Read the model definition and answer for the solid it produces. Units are mm, in the model's axes. Face numbers are marked on the shaded views. A direction names the side the tool comes from. Give positions to 0.01 mm unless a question says otherwise; leave off trailing zeros. Order: outer loops, then holes, each group sorted by start corner. A loop starts at its lowest first (then second) coordinate and runs counter-clockwise, first axis right, second up. Notation, with made-up numbers: (-15, 56) - (-4, 56) arc R35 ccw to (-4, 89) - close; hole circle Ø5 at (14.25, 83.5). An arc over 180 degrees is marked (long way). Write each question's results on one line, items separated by ' | '. Start each with the question number.
Q1. Find the intervals of material crossed by line 1 along Y through (x, z) = (5, 11); line 2 along X through (y, z) = (-0.3, 0); line 3 along X through (y, z) = (-0.15, -13.25), in increasing order. Write a range as from..to.
Q2. Find section B-B on x = 11.25. Give the vertices of the cut face in (y, z), and give its area (3 significant figures).
Q3. Flat-ended cylindrical pins translate along their axes: P1, Ø13, axis at y = 20.5, z = -6.5, coming from the +X side; P2, Ø10, axis at x = 10.5, z = 4, coming from the +Y side. Find the tip coordinate at first contact, or state that the pin passes through.
Q4. Find section A-A on z = 0. Give the vertices of the cut face in (x, y), and give its area (3 significant figures).
Q5. A tool of negligible diameter and unlimited length cuts with its end or side. For the marked faces 1 and 2, from which of +Z, -Z, +X, -X, +Y, -Y can it reach the whole face along a straight path? Write none if from no direction.
Q6. Find section C-C on z = -13.25. Give the vertices of the cut face in (x, y).
Q7. Find section D-D on y = 19. Give the vertices of the cut face in (x, z).
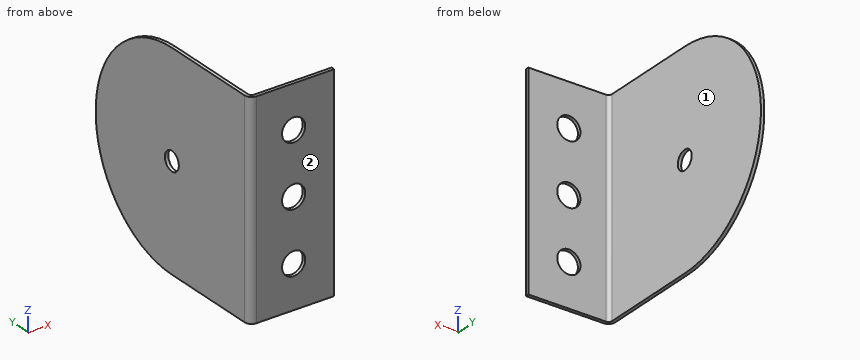
from build123d import *

# Parameters (mm, degrees)
SKETCH1_R                  = 2.5
SKETCH1_R_2                = 2.06
BASE_FLANGE3_DEPTH         = 0.7366
SKETCHED_START             = -43
SKETCHED_BEND1_OUTLINE_W   = 0.7366
SKETCHED_BEND1_OUTLINE_H   = 45
SKETCHED_BEND1_DEPTH       = 44.914756568
SKETCHED_START_2           = 2.495963432
SKETCHED_BEND1_2_OUTLINE_R = 2.06
SKETCHED_BEND1_2_DEPTH     = 0.004036568
SKETCHED_START_3           = 1.7634
SKETCHED_BEND1_3_OUTLINE_R = 2.06
SKETCHED_BEND1_3_DEPTH     = 1.4732
SKETCHED_START_4           = -23
SKETCHED_BEND1_4_DEPTH     = 46


with BuildPart() as part:
    # Base-Flange3: sheet metal written as solids
    # Sketch1 → Base-Flange3 (new body)
    with BuildSketch(Plane(origin=(0, 0, 0), x_dir=(1, 0, 0), z_dir=(0, 1, 0))):
        with BuildLine():
            Line((-20, 22.5), (20, 22.5))
            Line((20, 22.5), (20, -22.5))
            Line((20, -22.5), (-20, -22.5))
            ThreePointArc((-20, -22.5), (-42.5, 0), (-20, 22.5))
        make_face()
        with Locations(Location((11.25, -13.25, 0), (0, 0, 270))):
            Circle(SKETCH1_R, mode=Mode.SUBTRACT)
        with Locations(Location((11.25, 13.25, 0), (0, 0, 270))):
            Circle(SKETCH1_R, mode=Mode.SUBTRACT)
        with Locations(Location((11.25, 0, 0), (0, 0, 270))):
            Circle(SKETCH1_R, mode=Mode.SUBTRACT)
        with Locations(Location((-20, 0, 0), (0, 0, 270))):
            Circle(SKETCH1_R_2, mode=Mode.SUBTRACT)
    extrude(amount=-BASE_FLANGE3_DEPTH)

    # Sketched Bend1: read off the stored shape, not the designer's step
    # Sketched Bend1 outline → Sketched Bend1 (cut)
    with BuildSketch(Plane.YZ.offset(SKETCHED_START)):
        with Locations((-0.3683, 0)):
            Rectangle(SKETCHED_BEND1_OUTLINE_W, SKETCHED_BEND1_OUTLINE_H)
    extrude(amount=SKETCHED_BEND1_DEPTH, mode=Mode.SUBTRACT)

    # Sketched Bend1 2 outline → Sketched Bend1 2 (add)
    with BuildSketch(Plane.YZ.offset(SKETCHED_START_2)):
        with BuildLine():
            ThreePointArc((22.237627139, -22.5), (44.737627139, 0), (22.237627139, 22.5))
            Line((22.237627139, 22.5), (0, 22.5))
            Line((0, 22.5), (0, -22.5))
            Line((0, -22.5), (22.237627139, -22.5))
        make_face()
        with Locations((22.237627139, 0)):
            Circle(SKETCHED_BEND1_2_OUTLINE_R, mode=Mode.SUBTRACT)
    extrude(amount=SKETCHED_BEND1_2_DEPTH)

    # Sketched Bend1 3 outline → Sketched Bend1 3 (add)
    with BuildSketch(Plane.YZ.offset(SKETCHED_START_3)):
        with BuildLine():
            ThreePointArc((22.237627139, -22.5), (44.737627139, 0), (22.237627139, 22.5))
            Line((22.237627139, 22.5), (0, 22.5))
            Line((0, 22.5), (0, -22.5))
            Line((0, -22.5), (22.237627139, -22.5))
        make_face()
        with Locations((22.237627139, 0)):
            Circle(SKETCHED_BEND1_3_OUTLINE_R, mode=Mode.SUBTRACT)
    extrude(amount=SKETCHED_BEND1_3_DEPTH)

    # Sketched Bend1 4 outline → Sketched Bend1 4 (cut)
    with BuildSketch(Plane.XY.offset(SKETCHED_START_4)):
        with BuildLine():
            Line((2.5, 46), (2.5, 0.7366))
            ThreePointArc((2.5, 0.7366), (2.715745145, 0.215745145), (3.2366, 0))
            Line((3.2366, 0), (3.2366, 46))
            Line((3.2366, 46), (2.5, 46))
        make_face()
        with BuildLine():
            Line((1.7634, 0.7366), (1.763399995, 46))
            Line((1.763399995, 46), (0, 46))
            Line((0, 46), (0, 0))
            Line((0, 0), (1.914756568, 0))
            Line((1.914756568, 0), (1.914756568, -2))
            Line((1.914756568, -2), (5, -2))
            Line((5, -2), (5, -0.7366))
            Line((5, -0.7366), (3.2366, -0.7366))
            ThreePointArc((3.2366, -0.7366), (2.19489029, -0.30510971), (1.7634, 0.7366))
        make_face()
    extrude(amount=SKETCHED_BEND1_4_DEPTH, mode=Mode.SUBTRACT)


solid = part.part
Working result:
1) line 1: -0.74..0 | line 2: 2.19..8.75, 13.75..20 | line 3: 2.06..8.75, 13.75..20
2) outline: (-0.74, -22.5) - (0, -22.5) - (0, -15.75) - (-0.74, -15.75) - close; (-0.74, -10.75) - (0, -10.75) - (0, -2.5) - (-0.74, -2.5) - close; (-0.74, 2.5) - (0, 2.5) - (0, 10.75) - (-0.74, 10.75) - close; (-0.74, 15.75) - (0, 15.75) - (0, 22.5) - (-0.74, 22.5) - close | area: 22.1 mm²
3) P1: x = 2.5 | P2: y = 0
4) outline: (1.76, 0.74) arc R1.47 ccw to (3.24, -0.74) - (8.75, -0.74) - (8.75, 0) - (3.24, 0) arc R0.74 cw to (2.5, 0.74) - (2.5, 20.18) - (1.76, 20.18) - close; (1.76, 24.3) - (2.5, 24.3) - (2.5, 44.74) - (1.76, 44.74) - close; (13.75, -0.74) - (20, -0.74) - (20, 0) - (13.75, 0) - close | area: 39.3 mm²
5) face 1: +Z, -Z, +X, +Y | face 2: +Z, -Z, +X, -X, -Y
6) outline: (1.76, 0.74) arc R1.47 ccw to (3.24, -0.74) - (8.75, -0.74) - (8.75, 0) - (3.24, 0) arc R0.74 cw to (2.5, 0.74) - (2.5, 40.42) - (1.76, 40.42) - close; (13.75, -0.74) - (20, -0.74) - (20, 0) - (13.75, 0) - close
7) outline: (1.76, -22.5) - (2.5, -22.5) - (2.5, 22.5) - (1.76, 22.5) - close
